```python
from build123d import *

# Parameters (mm, degrees)
ESQUISSE1_W             = 222
ESQUISSE1_H             = 355.5
BOSS_EXTRU_1_DEPTH      = 3
ESQUISSE2_R             = 2
ESQUISSE2_W             = 15
ESQUISSE2_H             = 6
ENL_V_MAT_EXTRU_1_DEPTH = 3
ESQUISSE3_R             = 2
ESQUISSE3_W             = 12
ESQUISSE3_H             = 6
ENL_V_MAT_EXTRU_2_DEPTH = 3
ESQUISSE4_R             = 2
ESQUISSE4_W             = 202
ESQUISSE4_H             = 250
ENL_V_MAT_EXTRU_3_DEPTH = 3


with BuildPart() as part:
    # Esquisse1 → Boss.-Extru.1 (new body)
    with BuildSketch(Plane.XY):
        with Locations((61.472433281, -103.842323651)):
            Rectangle(ESQUISSE1_W, ESQUISSE1_H)
    extrude(amount=BOSS_EXTRU_1_DEPTH)

    # Esquisse2 → Enlèv. mat.-Extru.1 (cut)
    with BuildSketch(Plane.XY.offset(3)):
        with Locations((61.472433281, 70.907676349)):
            Circle(ESQUISSE2_R)
        with Locations(Location((61.472433281, -278.592323651, 0), (0, 0, 180))):
            Circle(ESQUISSE2_R)
        with Locations((8.972433281, 70.907676349)):
            Rectangle(ESQUISSE2_W, ESQUISSE2_H)
        with Locations((83.972433281, 70.907676349)):
            Rectangle(ESQUISSE2_W, ESQUISSE2_H)
        with Locations((143.972433281, 70.907676349)):
            Rectangle(ESQUISSE2_W, ESQUISSE2_H)
        with Locations((113.972433281, 70.907676349)):
            Rectangle(ESQUISSE2_W, ESQUISSE2_H)
        with Locations((-21.027566719, 70.907676349)):
            Rectangle(ESQUISSE2_W, ESQUISSE2_H)
        with Locations((38.972433281, 70.907676349)):
            Rectangle(ESQUISSE2_W, ESQUISSE2_H)
        with Locations((38.972433281, -278.592323651)):
            Rectangle(ESQUISSE2_W, ESQUISSE2_H)
        with Locations((-21.027566719, -278.592323651)):
            Rectangle(ESQUISSE2_W, ESQUISSE2_H)
        with Locations((8.972433281, -278.592323651)):
            Rectangle(ESQUISSE2_W, ESQUISSE2_H)
        with Locations((113.972433281, -278.592323651)):
            Rectangle(ESQUISSE2_W, ESQUISSE2_H)
        with Locations((143.972433281, -278.592323651)):
            Rectangle(ESQUISSE2_W, ESQUISSE2_H)
        with Locations((83.972433281, -278.592323651)):
            Rectangle(ESQUISSE2_W, ESQUISSE2_H)
    extrude(amount=-ENL_V_MAT_EXTRU_1_DEPTH, mode=Mode.SUBTRACT)

    # Esquisse3 → Enlèv. mat.-Extru.2 (cut)
    with BuildSketch(Plane.XY.offset(3)):
        with Locations((7.472433281, -205.092323651)):
            Circle(ESQUISSE3_R)
        with Locations(Location((115.472433281, -205.092323651, 0), (0, 0, 180))):
            Circle(ESQUISSE3_R)
        with Locations((49.472433281, -205.092323651)):
            Rectangle(ESQUISSE3_W, ESQUISSE3_H)
        with Locations((22.472433281, -205.092323651)):
            Rectangle(ESQUISSE3_W, ESQUISSE3_H)
        with Locations((-7.527566719, -205.092323651)):
            Rectangle(ESQUISSE3_W, ESQUISSE3_H)
        with Locations((-34.527566719, -205.092323651)):
            Rectangle(ESQUISSE3_W, ESQUISSE3_H)
        with Locations((157.472433281, -205.092323651)):
            Rectangle(ESQUISSE3_W, ESQUISSE3_H)
        with Locations((130.472433281, -205.092323651)):
            Rectangle(ESQUISSE3_W, ESQUISSE3_H)
        with Locations((100.472433281, -205.092323651)):
            Rectangle(ESQUISSE3_W, ESQUISSE3_H)
        with Locations((73.472433281, -205.092323651)):
            Rectangle(ESQUISSE3_W, ESQUISSE3_H)
    extrude(amount=-ENL_V_MAT_EXTRU_2_DEPTH, mode=Mode.SUBTRACT)

    # Esquisse4 → Enlèv. mat.-Extru.3 (cut)
    with BuildSketch(Plane.XY.offset(3)):
        with Locations((-44.527566719, -187.092323651)):
            Circle(ESQUISSE4_R)
        with Locations((-34.527566719, -197.092323651)):
            Circle(ESQUISSE4_R)
        with Locations(Location((157.472433281, -197.092323651, 0), (0, 0, 180))):
            Circle(ESQUISSE4_R)
        with Locations(Location((167.472433281, -187.092323651, 0), (0, 0, 180))):
            Circle(ESQUISSE4_R)
        with Locations((167.472433281, 52.907676349)):
            Circle(ESQUISSE4_R)
        with Locations((157.472433281, 62.907676349)):
            Circle(ESQUISSE4_R)
        with Locations(Location((-34.527566719, 62.907676349, 0), (0, 0, 180))):
            Circle(ESQUISSE4_R)
        with Locations(Location((-44.527566719, 52.907676349, 0), (0, 0, 180))):
            Circle(ESQUISSE4_R)
        with Locations((-44.527566719, -67.092323651)):
            Circle(ESQUISSE4_R)
        with Locations((167.472433281, -67.092323651)):
            Circle(ESQUISSE4_R)
        with Locations((61.472433281, 62.907676349)):
            Circle(ESQUISSE4_R)
        with Locations((61.472433281, -197.092323651)):
            Circle(ESQUISSE4_R)
        with Locations((61.472433281, -67.092323651)):
            Rectangle(ESQUISSE4_W, ESQUISSE4_H)
    extrude(amount=-ENL_V_MAT_EXTRU_3_DEPTH, mode=Mode.SUBTRACT)


solid = part.part
```
Source: CAD feature listing. Evaluate the final solid. Frame: model axes, mm. Round coordinates to 2 decimals unless told otherwise and drop trailing zeros. Write each loop counter-clockwise with the first axis right and the second up, starting at its lowest first coordinate (ties: lowest second). Pieces come first, ordered by that corner, then holes. Notation, with made-up numbers: M 23.5,81 L 62.5,81 A9 cw 62.5,95 Z; hole C -40,70.25 d11. An arc over 180 degrees is marked long. Use CSV: the item, a comma, the result in double quotes. Start each with the question number.
Q1. Cut plane B-B on x = 143. Output: boundary loops of the cut face in (y, z), plus the area to 4 significant figures.
Q2. First-contact query: P1, Ø1.5, axis at x = 109, z = 2, coming from the -Y side; P2, Ø1.5, axis at x = 84.5, z = 2, coming from the +Y side; P3, Ø3.5, axis at x = -44.53, y = 52.91, coming from the +Z side. Flat tips, straight axial feed; report the tip coordinate or a pass-through.
Q3. Cut plane A-A on y = -173.5. Output: boundary loops of the cut face in (x, z).
Q4. Line query: line 1 (Y direction, x = -2, z = 0.8); line 2 (X direction, y = -171.5, z = 1.6); line 3 (Y direction, x = 2, z = 2.8). Output: solid intervals per line, ascending. Write a range as from..to.
Q5. Cut plane C-C on z = 1.3. Count the separate pieces of the cut face and the enclosed holes in it, plus the area to 3 significant figures.
Results found:
1,outline,"M -275.59,0 L -192.09,0 L -192.09,3 L -275.59,3 Z; M 57.91,0 L 67.91,0 L 67.91,3 L 57.91,3 Z"
1,area,"280.5 mm^2"
2,P1,"y = -275.59"
2,P2,"y = 67.91"
2,P3,"through"
3,outline,"M -49.53,0 L -39.53,0 L -39.53,3 L -49.53,3 Z; M 162.47,0 L 172.47,0 L 172.47,3 L 162.47,3 Z"
4,line 1,"-281.59..-208.09, -202.09..-192.09, 57.91..73.91"
4,line 2,"-49.53..-39.53, 162.47..172.47"
4,line 3,"-275.59..-192.09, 57.91..67.91"
5,separate pieces,"1"
5,enclosed holes,"25"
5,area,"26,600 mm^2"
